from build123d import *

# Parameters (mm, degrees)
SKETCH001_W     = 120
SKETCH001_H     = 90
PAD_DEPTH       = 2
SKETCH_W        = 120
SKETCH_H        = 90
SKETCH_W_2      = 116
SKETCH_H_2      = 86
PAD001_DEPTH    = 47
SKETCH002_W     = 15
SKETCH002_H     = 16
SKETCH002_W_2   = 18.55
SKETCH002_H_2   = 15.2
POCKET_DEPTH    = 5
SKETCH003_R     = 3.75
POCKET001_DEPTH = 5
POCKET002_DEPTH = 5


with BuildPart() as part:
    # Sketch001 → Pad (new body)
    with BuildSketch(Plane.XY):
        with Locations((60, 45)):
            Rectangle(SKETCH001_W, SKETCH001_H)
    extrude(amount=PAD_DEPTH)

    # Sketch (on Face6 of Pad) → Pad001 (join)
    with BuildSketch(Plane.XY.offset(2)):
        with Locations((60, 45)):
            Rectangle(SKETCH_W, SKETCH_H)
        with Locations((60, 45)):
            Rectangle(SKETCH_W_2, SKETCH_H_2, mode=Mode.SUBTRACT)
    extrude(amount=PAD001_DEPTH)

    # Sketch002 (on Face8 of Pad001) → Pocket (cut)
    with BuildSketch(Plane.YZ.offset(120)):
        with Locations((11.5, 14.7)):
            Rectangle(SKETCH002_W, SKETCH002_H)
        with Locations((29.5, 14.7)):
            Rectangle(SKETCH002_W, SKETCH002_H)
        with Locations((48.275, 13.1)):
            Rectangle(SKETCH002_W_2, SKETCH002_H_2)
    extrude(amount=-POCKET_DEPTH, mode=Mode.SUBTRACT)

    # Sketch003 (on Face5 of Pocket) → Pocket001 (cut)
    with BuildSketch(Plane.XZ):
        with Locations((86, 9.3)):
            Circle(SKETCH003_R)
        with BuildLine():
            ThreePointArc((40.2, 10.65), (37.45, 7.9), (40.2, 5.15))
            Line((40.2, 5.15), (46.2, 5.15))
            ThreePointArc((46.2, 5.15), (48.95, 7.9), (46.2, 10.65))
            Line((40.2, 10.65), (46.2, 10.65))
        make_face()
        with BuildLine():
            Line((53.8, 10), (62.3, 10))
            Line((62.3, 10), (62.3, 7))
            ThreePointArc((60.55, 5.25), (61.787437, 5.762563), (62.3, 7))
            Line((60.55, 5.25), (55.55, 5.25))
            ThreePointArc((53.8, 7), (54.312563, 5.762563), (55.55, 5.25))
            Line((53.8, 7), (53.8, 10))
        make_face()
        with BuildLine():
            Line((67.2, 10), (75.7, 10))
            Line((75.7, 10), (75.7, 7))
            ThreePointArc((73.95, 5.25), (75.187437, 5.762563), (75.7, 7))
            Line((73.95, 5.25), (68.95, 5.25))
            ThreePointArc((67.2, 7), (67.712563, 5.762563), (68.95, 5.25))
            Line((67.2, 7), (67.2, 10))
        make_face()
    extrude(amount=-POCKET001_DEPTH, mode=Mode.SUBTRACT)

    # Sketch007 (on Face27 of Pocket001) → Pocket002 (cut)
    with BuildSketch(Plane(origin=(0, 90, 0), x_dir=(-1, 0, 0), z_dir=(0, 1, 0))):
        with BuildLine():
            ThreePointArc((-64, 10), (-65, 9), (-64, 8))
            Line((-64, 8), (-61.5, 8))
            ThreePointArc((-61.5, 8), (-60.5, 9), (-61.5, 10))
            Line((-64, 10), (-61.5, 10))
        make_face()
        with BuildLine():
            ThreePointArc((-56.5, 10), (-57.5, 9), (-56.5, 8))
            Line((-56.5, 8), (-54, 8))
            ThreePointArc((-54, 8), (-53, 9), (-54, 10))
            Line((-56.5, 10), (-54, 10))
        make_face()
        with BuildLine():
            ThreePointArc((-49, 10), (-50, 9), (-49, 8))
            Line((-49, 8), (-46.5, 8))
            ThreePointArc((-46.5, 8), (-45.5, 9), (-46.5, 10))
            Line((-49, 10), (-46.5, 10))
        make_face()
        with BuildLine():
            ThreePointArc((-41.5, 10), (-42.5, 9), (-41.5, 8))
            Line((-41.5, 8), (-39, 8))
            ThreePointArc((-39, 8), (-38, 9), (-39, 10))
            Line((-41.5, 10), (-39, 10))
        make_face()
        with BuildLine():
            ThreePointArc((-34, 10), (-35, 9), (-34, 8))
            Line((-34, 8), (-31.5, 8))
            ThreePointArc((-31.5, 8), (-30.5, 9), (-31.5, 10))
            Line((-34, 10), (-31.5, 10))
        make_face()
        with BuildLine():
            ThreePointArc((-26.5, 10), (-27.5, 9), (-26.5, 8))
            Line((-26.5, 8), (-24, 8))
            ThreePointArc((-24, 8), (-23, 9), (-24, 10))
            Line((-26.5, 10), (-24, 10))
        make_face()
        with BuildLine():
            ThreePointArc((-19, 10), (-20, 9), (-19, 8))
            Line((-19, 8), (-16.5, 8))
            ThreePointArc((-16.5, 8), (-15.5, 9), (-16.5, 10))
            Line((-19, 10), (-16.5, 10))
        make_face()
        with BuildLine():
            ThreePointArc((-11.5, 10), (-12.5, 9), (-11.5, 8))
            Line((-11.5, 8), (-9, 8))
            ThreePointArc((-9, 8), (-8, 9), (-9, 10))
            Line((-11.5, 10), (-9, 10))
        make_face()
    extrude(amount=-POCKET002_DEPTH, mode=Mode.SUBTRACT)


solid = part.part
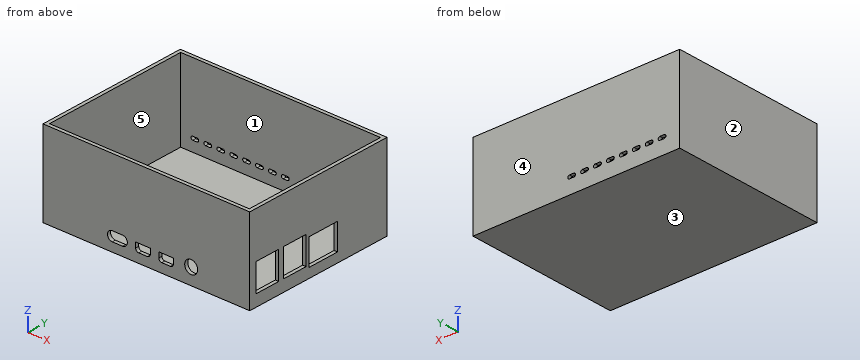
Geometry: final body of the model. Coordinates: model frame, mm. Face numbers are marked on the shaded views. A direction names the side the tool comes from. Round coordinates to 2 decimals unless told otherwise and drop trailing zeros. Loops run counter-clockwise (first coordinate to the right, second up) from the corner with the lowest first, then second, coordinate; pieces in that order, holes last. Notation, with made-up numbers: M 79,35.5 L 118,35.5 A22 ccw 118,73.5 Z; hole C -26.5,-23.75 d4. An arc over 180 degrees is marked long. One line per question, with ' | ' between items.
(1) Cut plane B-B on z = 15. Return the cut outline in (x, y).
Check result:
outline: M 0,0 L 120,0 L 120,4 L 118,4 L 118,2 L 2,2 L 2,88 L 118,88 L 118,57.55 L 120,57.55 L 120,90 L 0,90 Z; M 118,19 L 120,19 L 120,22 L 118,22 Z; M 118,37 L 120,37 L 120,39 L 118,39 Z
(2) Access query for the marked faces 4 and 5. Directions: +Z, -Z, +X, -X, +Y, -Y. A direction counts if a zero-diameter tool reaches every point of the face in a straight line with its end or side. Return the directions, or none.
Check result:
face 4: +Z, -Z, +X, -X, +Y | face 5: +Z
(3) Cut plane C-C on x = 86. Return the cut outline in (y, z), plus the area to 3 significant figures.
Check result:
outline: M 0,0 L 90,0 L 90,49 L 88,49 L 88,2 L 2,2 L 2,5.55 L 0,5.55 Z; M 0,13.05 L 2,13.05 L 2,49 L 0,49 Z | area: 353 mm2
(4) Contact query for flat-ended pins moving along their axis: P1, Ø1.5, axis at x = 22, y = 16.5, coming from the -Z side; P2, Ø12, axis at x = 88.5, y = 57, coming from the +Z side. Output: stop coordinate, or through.
Check result:
P1: stops at z = 0 | P2: stops at z = 2
(5) Cut plane A-A on z = 27. Return the cut outline in (x, y).
Check result:
outline: M 0,0 L 120,0 L 120,90 L 0,90 Z; hole M 2,2 L 118,2 L 118,88 L 2,88 Z
(6) Cut plane D-D on x = 109.5. Return the cut outline in (y, z), plus the area to 3 significant figures.
Check result:
outline: M 0,0 L 90,0 L 90,49 L 88,49 L 88,2 L 2,2 L 2,49 L 0,49 Z | area: 368 mm2
(7) Pull-direction query (X, two-part tool) for the marked faces 1, 2 and 3; classes: +X half, -X half, draft (parallel to the pull), parting line (faces both ways), or undercut.
Check result:
face 1: undercut | face 2: -X half | face 3: draft
(8) Material intervals for line 1 along X through (y, z) = (25.5, 26); line 2 along Z through (x, y) = (86, 1.5); line 3 along Y through (x, z) = (79.5, 41), sorted ascending. Write a range as from..to.
Check result:
line 1: x = 0..2, 118..120 | line 2: z = 0..5.55, 13.05..49 | line 3: y = 0..2, 88..90
